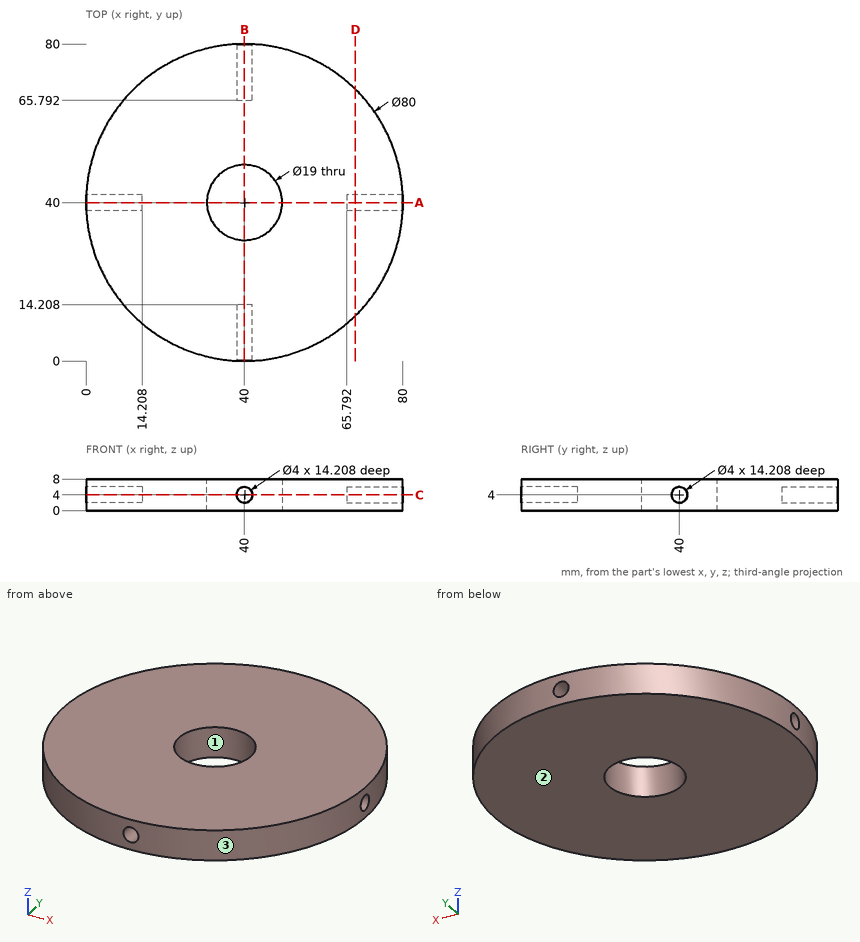
Print and shaded views of the part. All mm, measured from the part's lowest x, y and z. Coordinates: 2 decimals unless noted, no trailing zeros. Loops run counter-clockwise (first coordinate to the right, second up) from the corner with the lowest first, then second, coordinate; pieces in that order, holes last. Notation, with made-up numbers: (-3.5, 0) - (13.5, 0) arc R9 cw to (13.5, 15) - close; hole circle Ø3 at (54.25, -14). An arc over 180 degrees is marked (long way). Write item = value, one per line. Start each with the question number.
Item 1: Saw through at A-A, the plane y = 40. List the corners of the cut face in (x, z).
Item 2: Pull direction X, two halves, no side cores. Call the marked faces 1, 2 and 3: +X half, -X half, draft (parallel to the pull), parting line (faces both ways), or undercut.
Item 3: Saw through at D-D, the plane x = 68. List the corners of the cut face in (y, z), then the cut area to 3 significant figures.
Item 4: Wall check: probe 1 along Z at (x, y) = (40, 5); probe 2 along Y at (x, z) = (75, 2.5); probe 3 along X at (y, z) = (8, 5.75). Give the ranges that are in metal, low to high. Write a range as [from, to].
Item 5: Drop flat-ended pins along their axis: pin 1 Ø1.2 at (y, z) = (40, 4.5) entering from -X; pin 2 Ø3 at (y, z) = (40, 4) entering from +X; pin 3 Ø3.5 at (x, z) = (40, 4) entering from -Y. Give the stop position or say it passes through.
Item 6: Saw through at C-C, the plane z = 4. List the corners of the cut face in (x, y), then the cut area to 3 significant figures.
Answers:
q1.outline = (0, 0) - (30.5, 0) - (30.5, 8) - (0, 8) - (0, 6) - (14.21, 6) - (14.21, 2) - (0, 2) - close; (49.5, 0) - (80, 0) - (80, 2) - (65.79, 2) - (65.79, 6) - (80, 6) - (80, 8) - (49.5, 8) - close
q2.face_1 = undercut
q2.face_2 = draft
q2.face_3 = parting line
q3.outline = (11.43, 0) - (68.57, 0) - (68.57, 8) - (11.43, 8) - close; hole circle Ø4 at (40, 4)
q3.area = 444 mm2
q4.probe_1 = [0, 2], [6, 8]
q4.probe_2 = [20.64, 38.68], [41.32, 59.36]
q4.probe_3 = [16, 39.03], [40.97, 64]
q5.pin_1 = 14.21
q5.pin_2 = 65.79
q5.pin_3 = 14.21
q6.outline = (0.05, 38) arc R40 ccw to (38, 0.05) - (38, 14.21) - (42, 14.21) - (42, 0.05) arc R40 ccw to (79.95, 38) - (65.79, 38) - (65.79, 42) - (79.95, 42) arc R40 ccw to (42, 79.95) - (42, 65.79) - (38, 65.79) - (38, 79.95) arc R40 ccw to (0.05, 42) - (14.21, 42) - (14.21, 38) - close; hole circle Ø19 at (40, 40)
q6.area = 4,520 mm2
